Build history of the part. All positions in model axes, mm. Round coordinates to 2 decimals unless told otherwise and drop trailing zeros. Order: outer loops, then holes, each group sorted by start corner. A loop starts at its lowest first (then second) coordinate and runs counter-clockwise, first axis right, second up. Notation, with made-up numbers: M -32.5,68 L 13.5,68 A24 cw 13.5,92 Z; hole C 10.25,85.5 d8. An arc over 180 degrees is marked long. One line per question, with ' | ' between items. Start each with the question number.
from build123d import *

# Parameters (mm, degrees)
BOSS_EXTRUDE1_DEPTH     = 1.2
SKETCH3_R               = 1.2
CUT_EXTRUDE1_DEPTH      = 37.000138889
MIRROR2_COPY_1_SKETCH_R = 1.2
MIRROR2_COPY_1_DEPTH    = 37.000138889


with BuildPart() as part:
    # Sketch2 → Boss-Extrude1 (new, symmetric)
    with BuildSketch(Plane(origin=(0, 0, 0), x_dir=(1, 0, 0), z_dir=(0, 1, 0))):
        Polygon((-28, -14), (-28, 14), (-14.397156503, 22.5), (14.397156503, 22.5), (28, 14), (28, -14), (14.397156503, -22.5), (-14.397156503, -22.5), align=None)
    extrude(amount=BOSS_EXTRUDE1_DEPTH, both=True)

    # Sketch3 → Cut-Extrude1 (cut, through all)
    with BuildSketch(Plane(origin=(0, 1.2, 0), x_dir=(1, 0, 0), z_dir=(0, 1, 0))):
        with Locations(Location((-14.653288443, 19.8, 0), (0, 0, 270))):
            Circle(SKETCH3_R)
        with Locations(Location((-10.153288443, 19.8, 0), (0, 0, 270))):
            Circle(SKETCH3_R)
        with Locations(Location((-5.653288443, 19.8, 0), (0, 0, 270))):
            Circle(SKETCH3_R)
    cut_extrude1 = extrude(amount=-CUT_EXTRUDE1_DEPTH, mode=Mode.SUBTRACT)

    # Mirror1: Cut-Extrude1 across plane
    add(cut_extrude1.mirror(Plane(origin=(0, 0, 0), x_dir=(0, 0, 1), z_dir=(1, 0, 0))), mode=Mode.SUBTRACT)

    # Mirror2: Cut-Extrude1 across plane
    add(cut_extrude1.mirror(Plane.XY), mode=Mode.SUBTRACT)

    # Mirror2 copy 1 sketch → Mirror2 copy 1 (cut, through all)
    with BuildSketch(Plane(origin=(0, 1.2, 0), x_dir=(-1, 0, 0), z_dir=(0, 1, 0))):
        with Locations(Location((-14.653288443, 19.8, 0), (0, 0, 270))):
            Circle(MIRROR2_COPY_1_SKETCH_R)
        with Locations(Location((-10.153288443, 19.8, 0), (0, 0, 270))):
            Circle(MIRROR2_COPY_1_SKETCH_R)
        with Locations(Location((-5.653288443, 19.8, 0), (0, 0, 270))):
            Circle(MIRROR2_COPY_1_SKETCH_R)
    extrude(amount=-MIRROR2_COPY_1_DEPTH, mode=Mode.SUBTRACT)


solid = part.part
Item 1: Cut at B-B on y = 0.2. Count the separate pieces of the cut face and the enclosed holes in it, then the cut area to 3 significant figures.
Item 2: Cut at A-A on z = 19.8. Write the cut outline in (x, y).
Item 3: Flat gauge pins, fed straight in: pin 1 (1.9 mm diameter, centred on x = -14.65, z = 19.8, fed in from +Y); pin 2 (1 mm diameter, centred on x = 15.5, y = -0.5, fed in from -Z). Where does each tip first touch, or does it go through?
Item 4: Two-plate mould, pull along X, no slides. Class faces 1 (the face through (21.294, 0.017, 18.19)), 2 (the face through (-5.293, 0.017, 18.655)), 3 (the face through (0, 0, 22.5)): +X half, -X half, draft (parallel to the pull), parting line (faces both ways), or undercut.
Item 5: Wall check: line 1 along Z through (x, y) = (10, -0.15); line 2 along Z through (x, y) = (9.5, 0.9); line 3 along Z through (x, y) = (25.5, 0.55). Give the ranges that are in metal, low to high. Write a range as [from, to].
Results found:
1) separate pieces: 1 | enclosed holes: 12 | area: 2,230 mm^2
2) outline: M -18.72,-1.2 L -15.85,-1.2 L -15.85,1.2 L -18.72,1.2 Z; M -13.45,-1.2 L -11.35,-1.2 L -11.35,1.2 L -13.45,1.2 Z; M -8.95,-1.2 L -6.85,-1.2 L -6.85,1.2 L -8.95,1.2 Z; M -4.45,-1.2 L 4.45,-1.2 L 4.45,1.2 L -4.45,1.2 Z; M 6.85,-1.2 L 8.95,-1.2 L 8.95,1.2 L 6.85,1.2 Z; M 11.35,-1.2 L 13.45,-1.2 L 13.45,1.2 L 11.35,1.2 Z; M 15.85,-1.2 L 18.72,-1.2 L 18.72,1.2 L 15.85,1.2 Z
3) pin 1: passes through | pin 2: stops at z = -22.12
4) face 1: +X half | face 2: undercut | face 3: draft
5) line 1: z = [-22.5, -20.99], [-18.61, 18.61], [20.99, 22.5] | line 2: z = [-22.5, -20.81], [-18.79, 18.79], [20.81, 22.5] | line 3: z = [-15.56, 15.56]
